Geometry: see drawing. Coordinates: mm, zero at the bounding-box minimum. Coordinates: 2 decimals unless noted, no trailing zeros. Order: outer loops, then holes, each group sorted by start corner. A loop starts at its lowest first (then second) coordinate and runs counter-clockwise, first axis right, second up.
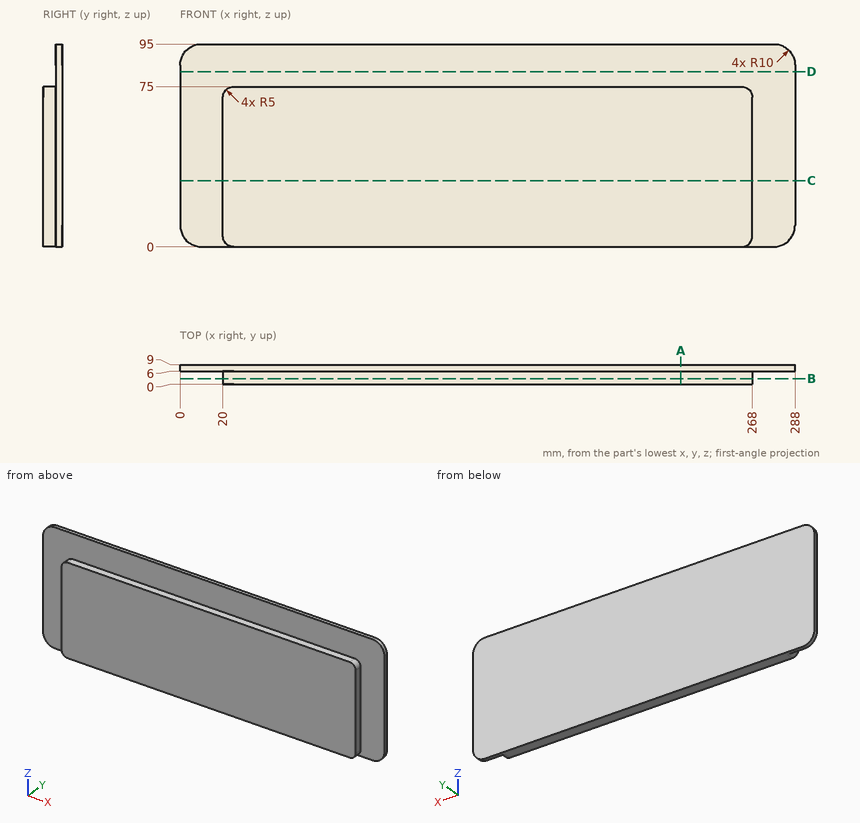
Q1. Material intervals for line 1 along X through (y, z) = (1.75, 26); line 2 along Z through (x, y) = (216.5, 2); line 3 along Y through (x, z) = (120.5, 83.5), sorted ascending.
Solutions:
line 1: x = 20 to 268
line 2: z = 0 to 75
line 3: y = 6 to 9
Q2. Section query D-D on z = 82. Output: boundary loops of the cut face in (x, y).
Solutions:
outline: (0, 6) - (288, 6) - (288, 9) - (0, 9) - close
Q3. Section query A-A on x = 234.5. Output: boundary loops of the cut face in (y, z), plus the area to 3 significant figures.
Solutions:
outline: (0, 0) - (9, 0) - (9, 95) - (6, 95) - (6, 75) - (0, 75) - close
area: 735 mm2
Q4. Pin query (flat end, axial travel): P1, Ø10, axis at x = 180.5, z = 63, coming from the -Y side; P2, Ø3, axis at y = 4, z = 16.5, coming from the -X side; P3, Ø1.5, axis at x = 190.5, z = 79.5, coming from the -Y side. Return the tip coordinate at first contact, or that it passes through.
Solutions:
P1: stops at y = 0
P2: stops at x = 20
P3: stops at y = 6
Q5. Section query C-C on z = 31. Output: boundary loops of the cut face in (x, y).
Solutions:
outline: (0, 6) - (20, 6) - (20, 0) - (268, 0) - (268, 6) - (288, 6) - (288, 9) - (0, 9) - close
Q6. Section query B-B on y = 2.5. Output: boundary loops of the cut face in (x, z).
Solutions:
outline: (20, 5) arc R5 ccw to (25, 0) - (263, 0) arc R5 ccw to (268, 5) - (268, 70) arc R5 ccw to (263, 75) - (25, 75) arc R5 ccw to (20, 70) - close
